Verification items for the finished model (mm, model axes). A direction names the side the tool comes from. Give positions to 0.01 mm unless a question says otherwise; leave off trailing zeros. Loops run counter-clockwise (first coordinate to the right, second up) from the corner with the lowest first, then second, coordinate; pieces in that order, holes last. Notation, with made-up numbers: (-29, 69.5) - (14, 69.5) arc R17 ccw to (14, 94.5) - close; hole circle Ø3 at (-3, 5). An arc over 180 degrees is marked (long way). One line per item, written item: value. Start each with the question number.
1. Scan lines: L1, parallel to Y at x = 113.5, z = 9.5; L2, parallel to X at y = -147.5, z = 4.25; L3, parallel to Y at x = 126.5, z = 3.5. Record each from-to range of solid material in increasing order. Write a range as [from, to].
2. Sectioned sample at C-C (z = 5). Count the separate pieces of the cut face and the enclosed holes in it, plus the area to 3 significant figures.
3. Mould release check, pull along Y, two halves, no side actions. Record for faces 3 (the cylindrical face through (95.42, -231.14, 3.93)), 4 (the cylindrical face through (96.35, -84.49, 3.93)), 5 (the cylindrical face through (136.194, -158.739, 3.925)), 6 (the flat face through (127, -223, -0.5)): pulls with the +Y half, pulls with the -Y half, needs draft (parallel to the pull), parting line crosses it, or undercut.
4. Gauge pin test, flat ends, axial feed: pin 1 (1.1 mm diameter, centred on x = 107, z = 9.5, fed in from +Y); pin 2 (4 mm diameter, centred on y = -186.5, z = 1.5, fed in from -X); pin 3 (1.6 mm diameter, centred on y = -91, z = -1.5, fed in from -X); pin 4 (3 mm diameter, centred on x = 129.16, y = -223.77, fed in from -Z). Record the tip position at first contact, or that the pin passes through.
5. Sectioned sample at B-B (y = -113.5). Record the cut outline in (x, z), plus the area to 3 significant figures.
6. Access from +Z, -Z, +X, -X, +Y, -Y to the whole of each face (thin tool, end or side, straight path). Record for faces 1 (the flat face through (61, -224, -0.5)), 2 (the cylindrical face through (127.42, -91.92, -1.26)).
7. Sectioned sample at A-A (x = 119). Record the cut outline in (y, z), plus the area to 3 significant figures.
from build123d import *
from build123d.topology import SkipClean

# Parameters (mm, degrees)
BOSS_EXTRU_1_DEPTH      = 10
COQUE3_START            = 62.865
COQUE3_OUTLINE_W        = 139.150614233
COQUE3_OUTLINE_H        = 10
COQUE3_DEPTH            = 66.018297978
COQUE3_2_DEPTH          = 66.018297978
COQUE3_START_2          = 132.445419336
COQUE3_3_OUTLINE_W      = 139.150614233
COQUE3_3_OUTLINE_H      = 10
COQUE3_3_DEPTH          = 0.002588282
COQUE3_4_DEPTH          = 10
COQUE3_START_3          = -2
COQUE3_5_DEPTH          = 12
COQUE3_6_DEPTH          = 2
ENL_V_START             = -10
ENL_V_MAT_EXTRU_4_DEPTH = 10
ESQUISSE5_R             = 1.8
BOSS_EXTRU_2_DEPTH      = 1.5
ESQUISSE6_R             = 1.8
ESQUISSE6_R_2           = 1.809836942
BOSS_EXTRU_3_DEPTH      = 1.5


with BuildPart() as part:
    # Model → Boss.-Extru.1 (new body)
    with BuildSketch(Plane.XY):
        with BuildLine():
            Line((62.865, -88.241118767), (128.905, -88.241118767))
            ThreePointArc((128.905, -88.241118767), (131.433274754, -89.251885129), (132.445419336, -91.779608456))
            Line((132.445419336, -91.779608456), (132.445419336, -223.843779))
            ThreePointArc((132.445419336, -223.843779), (131.447277728, -226.393080044), (128.898176953, -227.391733))
            Line((128.898176953, -227.391733), (62.865, -227.391733))
            ThreePointArc((62.865, -227.391733), (60.366111032, -226.356659298), (59.33103733, -223.85777033))
            Line((59.33103733, -223.85777033), (59.33103733, -91.775081437))
            ThreePointArc((59.33103733, -91.775081437), (60.366111032, -89.276192468), (62.865, -88.241118767))
        make_face()
    extrude(amount=BOSS_EXTRU_1_DEPTH)

    # Coque3: read off the stored shape, not the designer's step
    # Coque3 outline → Coque3 (cut)
    with BuildSketch(Plane.YZ.offset(COQUE3_START)):
        with Locations((-157.816425884, 5)):
            Rectangle(COQUE3_OUTLINE_W, COQUE3_OUTLINE_H)
    extrude(amount=COQUE3_DEPTH, mode=Mode.SUBTRACT)

    # Coque3 2 outline → Coque3 2 (add)
    with BuildSketch(Plane.YZ.offset(COQUE3_START)):
        Polygon((-227.391733, 10), (-229.391733, 10), (-229.391733, -2), (-86.241118767, -2), (-86.241118767, 10), (-88.241118767, 10), (-88.241118767, 0), (-227.391733, 0), align=None)
    extrude(amount=COQUE3_2_DEPTH)

    # Coque3 3 outline → Coque3 3 (add)
    with BuildSketch(Plane.YZ.offset(COQUE3_START_2)):
        with Locations((-157.816425884, 5)):
            Rectangle(COQUE3_3_OUTLINE_W, COQUE3_3_OUTLINE_H)
    extrude(amount=COQUE3_3_DEPTH)

    # Coque3 4 outline → Coque3 4 (cut)
    with BuildSketch(Plane.XY):
        with BuildLine():
            Line((62.865, -227.391733), (62.865, -88.241118767))
            ThreePointArc((62.865, -88.241118767), (60.366111032, -89.276192468), (59.33103733, -91.775081437))
            Line((59.33103733, -91.775081437), (59.33103733, -223.85777033))
            ThreePointArc((59.33103733, -223.85777033), (60.366111032, -226.356659298), (62.865, -227.391733))
        make_face()
        with BuildLine():
            Line((128.905, -88.241118767), (128.883297978, -88.241118767))
            Line((128.883297978, -88.241118767), (128.883297978, -227.391733))
            Line((128.883297978, -227.391733), (128.898176953, -227.391733))
            ThreePointArc((128.898176953, -227.391733), (131.447277728, -226.393080044), (132.445419336, -223.843779))
            Line((132.445419336, -223.843779), (132.445419336, -91.779608456))
            ThreePointArc((132.445419336, -91.779608456), (131.433274754, -89.251885129), (128.905, -88.241118767))
        make_face()
    extrude(amount=COQUE3_4_DEPTH, mode=Mode.SUBTRACT)

    # Coque3 5 outline → Coque3 5 (add)
    with SkipClean():  # the faces are left unmerged after this step: merging them gives an invalid solid
        with BuildSketch(Plane.XY.offset(COQUE3_START_3)):
            with BuildLine():
                ThreePointArc((62.865, -86.241118767), (58.951897469, -87.861978906), (57.33103733, -91.775081437))
                Line((57.33103733, -91.775081437), (57.33103733, -223.85777033))
                ThreePointArc((57.33103733, -223.85777033), (58.951897469, -227.770872861), (62.865, -229.391733))
                Line((62.865, -229.391733), (62.865, -227.391733))
                ThreePointArc((62.865, -227.391733), (60.366111032, -226.356659298), (59.33103733, -223.85777033))
                Line((59.33103733, -223.85777033), (59.33103733, -91.775081437))
                ThreePointArc((59.33103733, -91.775081437), (60.366111032, -89.276192468), (62.865, -88.241118767))
                Line((62.865, -88.241118767), (62.865, -86.241118767))
            make_face()
            with BuildLine():
                Line((128.883297978, -86.241118767), (128.883297978, -88.241118767))
                Line((128.883297978, -88.241118767), (128.905, -88.241118767))
                ThreePointArc((128.905, -88.241118767), (131.433274754, -89.251885129), (132.445419336, -91.779608456))
                Line((132.445419336, -91.779608456), (132.445419336, -223.843779))
                ThreePointArc((132.445419336, -223.843779), (131.447277728, -226.393080044), (128.898176953, -227.391733))
                Line((128.898176953, -227.391733), (128.883297978, -227.391733))
                Line((128.883297978, -227.391733), (128.883297978, -229.391733))
                Line((128.883297978, -229.391733), (128.863893168, -229.391733))
                ThreePointArc((128.863893168, -229.391733), (132.861554056, -227.807230841), (134.445419336, -223.80931758))
                Line((134.445419336, -223.80931758), (134.445419336, -91.8008272))
                ThreePointArc((134.445419336, -91.8008272), (132.847317492, -87.837500742), (128.883297978, -86.241118767))
            make_face()
        extrude(amount=COQUE3_5_DEPTH)
    add(part.part.scale(1), mode=Mode.REPLACE)  # the faces are merged on a copy

    # Coque3 6 outline → Coque3 6 (add)
    with BuildSketch(Plane.XY.offset(COQUE3_START_3)):
        with BuildLine():
            Line((62.865, -227.391733), (62.865, -88.241118767))
            ThreePointArc((62.865, -88.241118767), (60.366111032, -89.276192468), (59.33103733, -91.775081437))
            Line((59.33103733, -91.775081437), (59.33103733, -223.85777033))
            ThreePointArc((59.33103733, -223.85777033), (60.366111032, -226.356659298), (62.865, -227.391733))
        make_face()
        with BuildLine():
            Line((128.905, -88.241118767), (128.883297978, -88.241118767))
            Line((128.883297978, -88.241118767), (128.883297978, -227.391733))
            Line((128.883297978, -227.391733), (128.898176953, -227.391733))
            ThreePointArc((128.898176953, -227.391733), (131.447277728, -226.393080044), (132.445419336, -223.843779))
            Line((132.445419336, -223.843779), (132.445419336, -91.779608456))
            ThreePointArc((132.445419336, -91.779608456), (131.433274754, -89.251885129), (128.905, -88.241118767))
        make_face()
    extrude(amount=COQUE3_6_DEPTH)

    # Esquisse3 → Enlèv. mat.-Extru.4 (cut)
    with BuildSketch(Plane.XY.offset(ENL_V_START)):
        with BuildLine():
            Line((62.865, -88.241118767), (128.905, -88.241118767))
            ThreePointArc((128.905, -88.241118767), (131.433274754, -89.251885129), (132.445419336, -91.779608456))
            Line((132.445419336, -91.779608456), (132.445419336, -223.843779))
            ThreePointArc((132.445419336, -223.843779), (131.447277728, -226.393080044), (128.898176953, -227.391733))
            Line((128.898176953, -227.391733), (62.865, -227.391733))
            ThreePointArc((62.865, -227.391733), (60.366111032, -226.356659298), (59.33103733, -223.85777033))
            Line((59.33103733, -223.85777033), (59.33103733, -91.775081437))
            ThreePointArc((59.33103733, -91.775081437), (60.366111032, -89.276192468), (62.865, -88.241118767))
        make_face()
    extrude(amount=ENL_V_MAT_EXTRU_4_DEPTH, mode=Mode.SUBTRACT)

    # Esquisse5 → Boss.-Extru.2 (add)
    # profile 1 of 2: a face of its own
    with SkipClean():  # the faces are left unmerged after this step: merging them gives an invalid solid
        with BuildSketch(Plane(origin=(0, 0, -2), x_dir=(-1, 0, 0), z_dir=(0, 0, -1))):
            with BuildLine():
                Line((-125.967795303, -88.736416121), (-125.967795303, -87.927030419))
                Line((-125.967795303, -87.927030419), (-130.489542498, -87.7228715))
                Line((-130.489542498, -87.7228715), (-132.246258772, -88.33172327))
                Line((-132.246258772, -88.33172327), (-132.913956121, -88.736416121))
                Line((-132.913956121, -88.736416121), (-132.913956121, -95.223579528))
                Line((-132.913956121, -95.223579528), (-126.967795303, -95.223579528))
                ThreePointArc((-126.967795303, -95.223579528), (-126.260688522, -94.93068631), (-125.967795303, -94.223579528))
                Line((-125.967795303, -94.223579528), (-125.967795303, -88.736416121))
            make_face()
            with Locations((-129.134006805, -92.465411844)):
                Circle(ESQUISSE5_R, mode=Mode.SUBTRACT)
        # profile 2 of 2: a face of its own
        with BuildSketch(Plane(origin=(0, 0, -2), x_dir=(-1, 0, 0), z_dir=(0, 0, -1))):
            with BuildLine():
                Line((-65.780502675, -88.736416121), (-65.780502675, -87.927030419))
                Line((-65.780502675, -87.927030419), (-61.258755481, -87.7228715))
                Line((-61.258755481, -87.7228715), (-59.502039206, -88.33172327))
                Line((-59.502039206, -88.33172327), (-58.834341857, -88.736416121))
                Line((-58.834341857, -88.736416121), (-58.834341857, -95.223579528))
                Line((-58.834341857, -95.223579528), (-64.780502675, -95.223579528))
                ThreePointArc((-64.780502675, -95.223579528), (-65.487609456, -94.93068631), (-65.780502675, -94.223579528))
                Line((-65.780502675, -94.223579528), (-65.780502675, -88.736416121))
            make_face()
            with Locations((-62.957500414, -92.551168532)):
                Circle(ESQUISSE5_R, mode=Mode.SUBTRACT)
        extrude(amount=-BOSS_EXTRU_2_DEPTH)

    # Esquisse6 → Boss.-Extru.3 (add)
    # profile 1 of 2: a face of its own
    with BuildSketch(Plane(origin=(0, 0, -2), x_dir=(-1, 0, 0), z_dir=(0, 0, -1))):
        with BuildLine():
            Line((-133.339427004, -220.765848966), (-126.504202764, -220.765848966))
            ThreePointArc((-126.504202764, -220.765848966), (-125.797095983, -221.058742184), (-125.504202764, -221.765848966))
            Line((-125.504202764, -221.765848966), (-125.504202764, -228.064085465))
            Line((-125.504202764, -228.064085465), (-130.16804847, -228.064085465))
            Line((-130.16804847, -228.064085465), (-131.733408387, -227.250911482))
            Line((-131.733408387, -227.250911482), (-133.339427004, -225.177317824))
            Line((-133.339427004, -225.177317824), (-133.339427004, -220.765848966))
        make_face()
        with Locations((-129.160770539, -223.765453407)):
            Circle(ESQUISSE6_R, mode=Mode.SUBTRACT)
    # profile 2 of 2: a face of its own
    with BuildSketch(Plane(origin=(0, 0, -2), x_dir=(-1, 0, 0), z_dir=(0, 0, -1))):
        with BuildLine():
            Line((-58.389466164, -225.177317824), (-58.389466164, -220.765848966))
            Line((-58.389466164, -220.765848966), (-65.224690404, -220.765848966))
            ThreePointArc((-65.224690404, -220.765848966), (-65.931797185, -221.058742184), (-66.224690404, -221.765848966))
            Line((-66.224690404, -221.765848966), (-66.224690404, -228.064085465))
            Line((-66.224690404, -228.064085465), (-61.560844698, -228.064085465))
            Line((-61.560844698, -228.064085465), (-59.995484781, -227.250911482))
            Line((-59.995484781, -227.250911482), (-58.389466164, -225.177317824))
        make_face()
        with Locations((-63.12082636, -223.851047054)):
            Circle(ESQUISSE6_R_2, mode=Mode.SUBTRACT)
    extrude(amount=-BOSS_EXTRU_3_DEPTH)

    # Balayage1: sweep along a path in Esquisse7
    with BuildLine(Plane.XY.offset(5)) as balayage1_path:
        Line((128.942747104, -230.887624532), (62.83103733, -230.887624532))
        ThreePointArc((62.83103733, -230.887624532), (57.881289862, -228.837372001), (55.83103733, -223.887624532))
        Line((55.83103733, -223.887624532), (55.83103733, -91.741118767))
        ThreePointArc((55.83103733, -91.741118767), (57.881289862, -86.791371299), (62.83103733, -84.741118767))
        Line((62.83103733, -84.741118767), (128.942747104, -84.741118767))
        ThreePointArc((128.942747104, -84.741118767), (133.892494572, -86.791371299), (135.942747104, -91.741118767))
        Line((135.942747104, -91.741118767), (135.942747104, -223.887624532))
        ThreePointArc((135.942747104, -223.887624532), (133.892494572, -228.837372001), (128.942747104, -230.887624532))
    # Esquisse8 → Balayage1 (sweep)
    with BuildSketch(Plane(origin=(0, -155, 0), x_dir=(1, 0, 0), z_dir=(0, 1, 0))):
        with BuildLine():
            Line((57.33103733, 1.001505866), (57.33103733, -9.003220236))
            ThreePointArc((57.33103733, -9.003220236), (55.579057649, -4.000857185), (57.33103733, 1.001505866))
        make_face()
    sweep(path=balayage1_path.line)


solid = part.part
Results are:
1. L1: y = [-229.39, -227.39], [-88.24, -86.24]
1. L2: x = [55.58, 59.33], [132.45, 136.19]
1. L3: y = [-231.12, -227.39], [-88.24, -84.5]
2. separate pieces: 1
2. enclosed holes: 3
2. area: 1,590 mm^2
3. face 3: pulls with the -Y half
3. face 4: pulls with the +Y half
3. face 5: needs draft
3. face 6: undercut
4. pin 1: stops at y = -86.2
4. pin 2: stops at x = 55.59
4. pin 3: stops at x = 57.14
4. pin 4: passes through
5. outline: (57.33, -2) - (59.33, -2) - (59.33, 10) - (57.33, 10) - (57.33, 9) arc R8.02 ccw to (57.33, -1) - close; (132.45, -2) - (134.45, -2) - (134.45, -1) arc R8.02 ccw to (134.45, 9) - (134.45, 10) - (132.45, 10) - close
5. area: 71.9 mm^2
6. face 1: +Z
6. face 2: +Z, -Z
7. outline: (-229.39, -2) - (-227.39, -2) - (-227.39, 10) - (-229.39, 10) - (-229.39, 9) arc R8.02 ccw to (-229.39, -1) - close; (-88.24, -2) - (-86.24, -2) - (-86.24, -1) arc R8.02 ccw to (-86.24, 9) - (-86.24, 10) - (-88.24, 10) - close
7. area: 71.9 mm^2
